Autodesk Inventor part; units mm, degrees
ref_plane "YZ Plane" through (0, 0, 0) normal (1, 0, 0) x (0, 1, 0)
ref_plane "XZ Plane" through (0, 0, 0) normal (0, 1, 0) x (-1, 0, 0)
ref_plane "XY Plane" through (0, 0, 0) normal (0, 0, 1) x (1, 0, 0)
sketch "Sketch1" plane through (0, 0, 0) normal (0, 0, 1) x (1, 0, 0)
  line L0 (0, 0) -> (38.1, 0)
  line L1 (38.1, 0) -> (38.1, 31.75)
  line L2 (38.1, 31.75) -> (0, 31.75)
  line L3 (0, 31.75) -> (0, 0)
  dimension "d0" = 38.1
  dimension "d1" = 31.75
extrude "Extrusion1" add sketch "Sketch1" along normal blind 19.05
sketch "Sketch2" plane through (0, 0, 19.05) normal (0, 0, 1) x (1, 0, 0)
  line L0 (31.5532, 15.8754) -> (6.5532, 15.8754)
  line L1 (19.0532, 6.3754) -> (19.0532, 25.3754)
  line L2 (0, 31.75) -> (0, 0)
  line L3 (38.1, 0) -> (0, 0)
  line L4 (0, 0) -> (38.1, 0)
  line L5 (0, 31.75) -> (0, 0)
  point P0 (19.0532, 15.8754)
  point P1 (0, -6.35)
  point P2 (9.525, -9.525)
  dimension "d4" = 25
  dimension "d5" = 19
  dimension "d6" = 6.5532
  dimension "d7" = 6.3754
hole "Hole1" at (19.0532, 15.8754, 19.05) at (19.0532, 25.3754, 19.05) at (6.5532, 15.8754, 19.05) at (19.0532, 6.3754, 19.05) at (31.5532, 15.8754, 19.05) direction (0, 0, -1) diameter 3.4036 depth 32.0675
sketch "Sketch3" plane through (0, 0, 0) normal (0, 0, -1) x (-1, 0, 0)
  circle A0 centre (-19.0532, 6.3754) radius 1.7018
  circle A1 centre (-19.0532, 25.3754) radius 1.7018
  circle A2 centre (-19.0532, 15.8754) radius 1.7018
  circle A3 centre (-6.5532, 15.8754) radius 1.7018
  circle A4 centre (-31.5532, 15.8754) radius 1.7018
  line L0 (-38.1, 0) -> (-38.1, 31.75)
  line L1 (0, 0) -> (-38.1, 0)
  line L2 (0, 31.75) -> (0, 0)
  line L3 (-38.1, 31.75) -> (0, 31.75)
  circle A5 centre (-19.0532, 25.3754) radius 1.7018
  circle A6 centre (-19.0532, 6.3754) radius 1.7018
  circle A7 centre (-19.0532, 15.8754) radius 1.7018
  circle A8 centre (-19.0532, 15.8754) radius 5.5
  dimension "d34" = 11
hole "Hole2" at (19.0532, 15.8754, 0) at (19.0532, 25.3754, 0) at (31.5532, 15.8754, 0) at (6.5532, 15.8754, 0) at (19.0532, 6.3754, 0) direction (0, 0, 1) diameter 6.096 depth 16.002
chamfer "Chamfer1" distance 1.016 angle 45 5 edges at (19.0532, 8.0772, 16.002) (6.5532, 17.5772, 16.002) (19.0532, 17.5772, 16.002) (19.0532, 27.0772, 16.002) (31.5532, 17.5772, 16.002)
sketch "Sketch4" plane through (0, 0, 0) normal (0, -1, 0) x (1, 0, 0)
  line L0 (0, 0) -> (38.1, 0)
  line L1 (38.1, 0) -> (38.1, 19.05)
  line L2 (0, 19.05) -> (38.1, 19.05)
  line L3 (0, 0) -> (0, 19.05)
  line L4 (17.3514, 19.05) -> (20.755, 19.05)
  line L5 (19.0532, 19.05) -> (19.05, 0)
  point P0 (8.128, 9.525)
  point P1 (29.9752, 9.5213)
  point P2 (0, 9.525)
  dimension "d25" = 9.525
  dimension "d26" = 8.128
hole "Hole3" at (8.128, 0, 9.525) at (29.9752, 0, 9.5213) direction (0, 1, 0) diameter 7.112 depth 10.414
sketch "Sketch5" plane through (0, 0, 19.05) normal (0, 0, 1) x (1, 0, 0)
  circle A0 centre (19.0532, 15.8754) radius 1.7018
  circle A1 centre (19.0532, 15.8754) radius 6
  point P0 (0, 0)
  dimension "d35" = 12
extrude "Extrusion2" cut sketch "Sketch5" against normal blind 25.4
fillet "Fillet2" radius 6.35 2 edges at (0, 31.75, 9.525) (38.1, 31.75, 9.525)
properties part number "Motor Mounts"
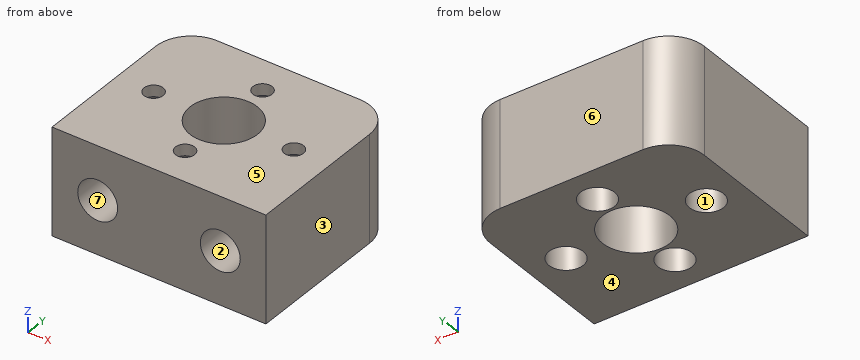
Read the model definition and answer for the solid it produces. Units are mm, in the model's axes. Face numbers are marked on the shaded views. A direction names the side the tool comes from. Give positions to 0.01 mm unless a question says otherwise; leave off trailing zeros. Write each loop counter-clockwise with the first axis right and the second up, starting at its lowest first coordinate (ties: lowest second). Pieces come first, ordered by that corner, then holes. Notation, with made-up numbers: M 17,76.25 L 73,76.25 A9 cw 73,93.25 Z; hole C 46,48 d2. An arc over 180 degrees is marked long. One line per item, written item: value. Start each with the question number.
(1) Find section A-A (x = 27). Determine the outline of the cut face in (y, z), plus the area to 3 significant figures.
(2) Find section C-C (y = 7.5). Give the number of separate pieces and of enclosed holes in the cut face, plus the area to 3 significant figures.
(3) Flat-ended cylindrical pins translate along their axes: pin 1 Ø3.5 at (x, z) = (8, 8) entering from -Y; pin 2 Ø3 at (x, y) = (7, 16) entering from -Z; pin 3 Ø5.5 at (x, y) = (19.05, 6.38) entering from -Z. Find the tip coordinate at first contact, or state that the pin passes through.
(4) Find section D-D (z = 7). Determine the outline of the cut face in (x, y), plus the area to 3 significant figures.
(5) Find section B-B (z = 2). Determine the outline of the cut face in (x, y).
(6) Determine the mould class of the marked faces 4, 5, 6 and 7 for opening direction Z: pulls with the +Z half, pulls with the -Z half, needs draft (parallel to the pull), parting line crosses it, or undercut.
(7) A tool of negligible diameter and unlimited length cuts with its end or side. For the marked faces 1, 2 and 3, from which of +Z, -Z, +X, -X, +Y, -Y can it reach the whole face along a straight path? Write none if from no direction.
(8) Find the intervals of material crossed by line 1 (X direction, y = 24, z = 12.75); line 2 (X direction, y = 4, z = 11.75); line 3 (X direction, y = 3, z = 7.75), in increasing order.
Results below:
1. outline: M 0,0 L 31.75,0 L 31.75,19.05 L 0,19.05 L 0,11.47 L 10.41,11.47 L 10.41,7.57 L 0,7.57 Z
1. area: 564 mm^2
2. separate pieces: 2
2. enclosed holes: 2
2. area: 547 mm^2
3. pin 1: stops at y = 10.41
3. pin 2: stops at z = 16.76
3. pin 3: stops at z = 16
4. outline: M 0,0 L 5.62,0 L 5.62,10.41 L 10.63,10.41 L 10.63,0 L 27.47,0 L 27.47,10.41 L 32.48,10.41 L 32.48,0 L 38.1,0 L 38.1,25.4 A6.35 ccw 31.75,31.75 L 6.35,31.75 A6.35 ccw 0,25.4 Z; hole C 6.55,15.88 d6.1; hole C 19.05,15.88 d12; hole C 19.05,6.38 d6.1; hole C 19.05,25.38 d6.1; hole C 31.55,15.88 d6.1
4. area: 858 mm^2
5. outline: M 0,0 L 38.1,0 L 38.1,25.4 A6.35 ccw 31.75,31.75 L 6.35,31.75 A6.35 ccw 0,25.4 Z; hole C 6.55,15.88 d6.1; hole C 19.05,15.88 d12; hole C 19.05,6.38 d6.1; hole C 19.05,25.38 d6.1; hole C 31.55,15.88 d6.1
6. face 4: pulls with the -Z half
6. face 5: pulls with the +Z half
6. face 6: needs draft
6. face 7: undercut
7. face 1: -Z
7. face 2: -Y
7. face 3: +Z, -Z, +X, +Y, -Y
8. line 1: x = 0 to 16.33, 21.77 to 38.1
8. line 2: x = 0 to 5.35, 10.9 to 17.14, 20.96 to 27.2, 32.75 to 38.1
8. line 3: x = 0 to 5.05, 11.21 to 26.89, 33.06 to 38.1
